Read the model definition and answer for the solid it produces. Units are mm, in the model's axes. A direction names the side the tool comes from. Give positions to 0.01 mm unless a question says otherwise; leave off trailing zeros. Order: outer loops, then holes, each group sorted by start corner. A loop starts at its lowest first (then second) coordinate and runs counter-clockwise, first axis right, second up. Notation, with made-up numbers: (-35.5, -20.5) - (-26.5, -20.5) arc R13 ccw to (-26.5, -5.5) - close; hole circle Ø10 at (4.25, 86). An arc over 180 degrees is marked (long way). Write each question's results on one line, items separated by ' | '. Start each with the question number.
Q1. For a pull along X with two mould halves and no side action, classify faces 4 (the face through (19, 4.965, 59)), 5 (the face through (-31, -24, 35)), 6 (the face through (31, -24, 35)) as +X half, -X half, draft (parallel to the pull), parting line (faces both ways), or undercut.
Q2. Find section C-C on z = 65. Give the vertices of the cut face in (x, y).
Q3. A tool of negligible diameter and unlimited length cuts with its end or side. For faces 1 (the face through (-25, 4, 35)), 2 (the face through (-15.98, 22.05, 8.97)), 3 (the face through (25, 5, 35)), from which of +Z, -Z, +X, -X, +Y, -Y can it reach the whole face along a straight path? Write none if from no direction.
Q4. Find section D-D on x = -19. Give the vertices of the cut face in (y, z), and give its area (3 significant figures).
Q5. Find the intervals of material crossed by line 1 along Z through (x, y) = (-19, 18); line 2 along Z through (x, y) = (-19, 12); line 3 along Y through (x, z) = (0, 24.5), in increasing order. Write a range as from..to.
Q6. Find section A-A on x = 0. Give the vertices of the cut face in (y, z).
Q7. Find section B-B on y = 6. Give the vertices of the cut face in (x, z).
Q8. Flat-ended cylindrical pins translate along their axes: P1, Ø3, axis at y = 4.5, z = 8, coming from the -X side; P2, Ø4, axis at x = 19.5, z = 59.5, coming from the +Y side; P3, Ø4, axis at y = -5.5, z = 15, coming from the +X side. Find the tip coordinate at first contact, or state that the pin passes through.
from build123d import *

# Parameters (mm, degrees)
SKETCH1_R           = 12.5
BOSS_EXTRUDE1_DEPTH = 70
SKETCH2_R           = 3.805013563
CUT_EXTRUDE1_DEPTH  = 23
SKETCH3_R           = 3.805013563
CUT_EXTRUDE2_DEPTH  = 12


with BuildPart() as part:
    # Sketch1 → Boss-Extrude1 (new body)
    with BuildSketch(Plane.XY):
        Polygon((25, -19.03462444), (31, -19.03462444), (31, -29.03462444), (-31, -29.03462444), (-31, -19.03462444), (-25, -19.03462444), (-25, 27.96537556), (25, 27.96537556), align=None)
        with Locations((0, 4.96537556)):
            Circle(SKETCH1_R, mode=Mode.SUBTRACT)
    extrude(amount=BOSS_EXTRUDE1_DEPTH)

    # Sketch2 → Cut-Extrude1 (cut)
    with BuildSketch(Plane(origin=(0, 27.96537556, 0), x_dir=(1, 0, 0), z_dir=(0, 1, 0))):
        with Locations(Location((19, -58.714630835, 0), (0, 0, 180))):
            Circle(SKETCH2_R)
        with Locations((-19, -58.714630835)):
            Circle(SKETCH2_R)
    extrude(amount=-CUT_EXTRUDE1_DEPTH, mode=Mode.SUBTRACT)

    # Sketch3 → Cut-Extrude2 (cut)
    with BuildSketch(Plane(origin=(0, 27.96537556, 0), x_dir=(1, 0, 0), z_dir=(0, 1, 0))):
        with Locations((19, -11.285369165)):
            Circle(SKETCH3_R)
        with Locations(Location((-19, -11.285369165, 0), (0, 0, 180))):
            Circle(SKETCH3_R)
    extrude(amount=-CUT_EXTRUDE2_DEPTH, mode=Mode.SUBTRACT)


solid = part.part
Working result:
1) face 4: undercut | face 5: -X half | face 6: +X half
2) outline: (-31, -29.03) - (31, -29.03) - (31, -19.03) - (25, -19.03) - (25, 27.97) - (-25, 27.97) - (-25, -19.03) - (-31, -19.03) - close; hole circle Ø25 at (0, 4.97)
3) face 1: +Z, -Z, -X, +Y | face 2: +Y | face 3: +Z, -Z, +X, +Y
4) outline: (-29.03, 0) - (27.97, 0) - (27.97, 7.48) - (15.97, 7.48) - (15.97, 15.09) - (27.97, 15.09) - (27.97, 54.91) - (4.97, 54.91) - (4.97, 62.52) - (27.97, 62.52) - (27.97, 70) - (-29.03, 70) - close | area: 3,720 mm²
5) line 1: 0..7.48, 15.09..54.91, 62.52..70 | line 2: 0..54.91, 62.52..70 | line 3: -29.03..-7.53, 17.47..27.97
6) outline: (-29.03, 0) - (-7.53, 0) - (-7.53, 70) - (-29.03, 70) - close; (17.47, 0) - (27.97, 0) - (27.97, 70) - (17.47, 70) - close
7) outline: (-25, 0) - (-12.46, 0) - (-12.46, 70) - (-25, 70) - close; (12.46, 0) - (25, 0) - (25, 70) - (12.46, 70) - close; hole circle Ø7.61 at (-19, 58.71); hole circle Ø7.61 at (19, 58.71)
8) P1: x = -25 | P2: y = 4.97 | P3: x = 25
